Model file for the job. Use its own axes, mm. Face numbers are marked on the shaded views. A direction names the side the tool comes from. Round coordinates to 2 decimals unless told otherwise and drop trailing zeros. Loops run counter-clockwise (first coordinate to the right, second up) from the corner with the lowest first, then second, coordinate; pieces in that order, holes last.
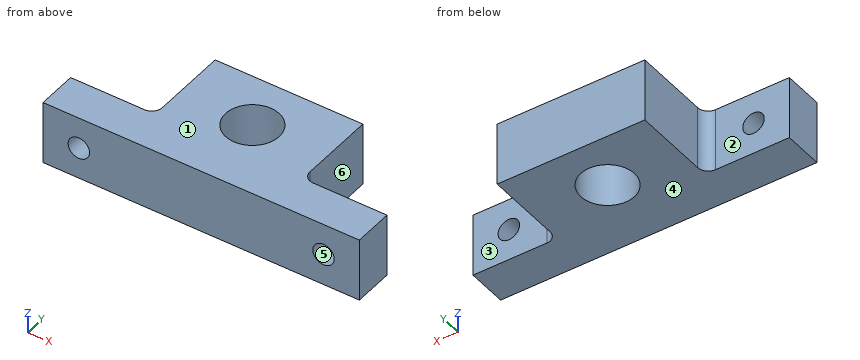
from build123d import *

# Parameters (mm, degrees)
BOSS_EXTRUDE1_DEPTH               = 30
F_1_1_0000_DOWEL_HOLE1_D          = 25.4
TAP_DRILL_FOR_M12X1_75_TAP1_D     = 10.2
TAP_DRILL_FOR_M12X1_75_TAP1_DEPTH = 30
TAP_DRILL_FOR_M12X1_75_TAP1_TIP   = 3.064389157


with BuildPart() as part:
    # Sketch1 → Boss-Extrude1 (new body)
    with BuildSketch(Plane.XY):
        with BuildLine():
            Line((-75, -23.452240915), (75, -23.452240915))
            Line((75, -23.452240915), (75, -4.569806156))
            Line((75, -4.569806156), (40, -4.569806156))
            ThreePointArc((40, -4.569806156), (36.464466094, -3.105340062), (35, 0.430193844))
            Line((35, 0.430193844), (35, 36.547759085))
            Line((35, 36.547759085), (-35, 36.547759085))
            Line((-35, 36.547759085), (-35, 0.430193844))
            ThreePointArc((-35, 0.430193844), (-36.464466094, -3.105340062), (-40, -4.569806156))
            Line((-40, -4.569806156), (-75, -4.569806156))
            Line((-75, -4.569806156), (-75, -23.452240915))
        make_face()
    extrude(amount=BOSS_EXTRUDE1_DEPTH)

    # 1 (1.0000) Dowel Hole1 (through all)
    with Locations(Plane.XY.offset(30)):
        with Locations((0, 11.547759085)):
            Hole(F_1_1_0000_DOWEL_HOLE1_D / 2)

    # Tap Drill for M12x1.75 Tap1
    with Locations(Plane(origin=(0, -4.569806156, 0), x_dir=(1, 0, 0), z_dir=(0, 1, 0))):
        with Locations((58, -15), (-58, -15)):
            Hole(TAP_DRILL_FOR_M12X1_75_TAP1_D / 2, depth=TAP_DRILL_FOR_M12X1_75_TAP1_DEPTH)
            with Locations((0, 0, -(TAP_DRILL_FOR_M12X1_75_TAP1_DEPTH + TAP_DRILL_FOR_M12X1_75_TAP1_TIP / 2))):  # 118° drill point
                Cone(0, TAP_DRILL_FOR_M12X1_75_TAP1_D / 2, TAP_DRILL_FOR_M12X1_75_TAP1_TIP, mode=Mode.SUBTRACT)


solid = part.part
Q1. Slice it at B-B on z = 15. Give the cut face in (x, y).
Q2. Probe line 1 (X direction, y = -16.5, z = 15.25); line 2 (Z direction, x = -58, y = -9); line 3 (Y direction, x = 0, z = 18.5). List the from-to ranges inside material, lowest first.
Q3. Slice it at D-D on y = -13. Give the cut face in (x, z), plus the area to 3 significant figures.
Q4. Pull direction Z, two halves, no side cores. Call the marked faces 4, 5 and 6: pulls with the +Z half, pulls with the -Z half, needs draft (parallel to the pull), parting line crosses it, or undercut.
Q5. Tool access for the marked faces 1, 2 and 3: list every direction of +Z, -Z, +X, -X, +Y, -Y with a clear straight run to the whole face (end or side of a thin tool).
Q6. Flat gauge pins, fed straight in: P1, Ø4, axis at y = 19, z = 7, coming from the -X side; P2, Ø9, axis at x = -51, z = 8.5, coming from the +Y side. Where does each tip first touch, or does it go through?
Q7. Slice it at A-A on x = 0. Give the cut face in (y, z), plus the area to 3 significant figures.
Q8. Slice it at C-C on y = 19.5. Give the cut face in (x, z).
Reply:
1. outline: (-75, -23.45) - (-63.1, -23.45) - (-63.1, -4.57) - (-75, -4.57) - close; (-52.9, -23.45) - (52.9, -23.45) - (52.9, -4.57) - (40, -4.57) arc R5 cw to (35, 0.43) - (35, 36.55) - (-35, 36.55) - (-35, 0.43) arc R5 cw to (-40, -4.57) - (-52.9, -4.57) - close; (63.1, -23.45) - (75, -23.45) - (75, -4.57) - (63.1, -4.57) - close; hole circle Ø25.4 at (0, 11.55)
2. line 1: x = -75 to -63.09, -52.91 to 52.91, 63.09 to 75
2. line 2: z = 0 to 9.9, 20.1 to 30
2. line 3: y = -23.45 to -1.15, 24.25 to 36.55
3. outline: (-75, 0) - (75, 0) - (75, 30) - (-75, 30) - close; hole circle Ø10.2 at (-58, 15); hole circle Ø10.2 at (58, 15)
3. area: 4,340 mm2
4. face 4: pulls with the -Z half
4. face 5: undercut
4. face 6: needs draft
5. face 1: +Z, +X, -X, +Y, -Y
5. face 2: +Z, -Z, -X, +Y
5. face 3: +Z, -Z, +X, +Y
6. P1: stops at x = -35
6. P2: stops at y = -4.57
7. outline: (-23.45, 0) - (-1.15, 0) - (-1.15, 30) - (-23.45, 30) - close; (24.25, 0) - (36.55, 0) - (36.55, 30) - (24.25, 30) - close
7. area: 1,040 mm2
8. outline: (-35, 0) - (-9.9, 0) - (-9.9, 30) - (-35, 30) - close; (9.9, 0) - (35, 0) - (35, 30) - (9.9, 30) - close
